The listing builds one solid part. Answer for the finished solid, in the listing's coordinates (mm). Face numbers are marked on the shaded views. A direction names the side the tool comes from. Coordinates: 2 decimals unless noted, no trailing zeros. Order: outer loops, then holes, each group sorted by start corner. A loop starts at its lowest first (then second) coordinate and runs counter-clockwise, first axis right, second up. Notation, with made-up numbers: (74, 27.25) -> (122, 27.25) arc R16 cw to (122, 56.25) -> close; hole circle Ø6 at (-22, -22.5). An arc over 180 degrees is marked (long way). Write each question's results on one line, items separated by ' | '. Start each with the question number.
(1) The part is cut by section A-A, the plane y = 49.5. Give the vertices of the cut face in (x, z) (3 decimals).
(2) Given pin 1 (4 mm diameter, centred on x = 12, z = 48.5, fed in from -Y); pin 2 (11 mm diameter, centred on y = -19.5, z = 8, fed in from +X) (3 decimals); pin 3 (5 mm diameter, centred on y = -28.5, z = 50.5, fed in from +X); pin 4 (14 mm diameter, centred on y = -17.5, z = 19.5, fed in from -X) (3 decimals), each flat-ended and moving along its own axis, determine where each tip first touches the part or whether it passes through.
(3) Determine the mould class of the marked faces 4, 5 and 6 for opening direction X: +X half, -X half, draft (parallel to the pull), parting line (faces both ways), or undercut.
(4) A tool of negligible diameter and unlimited length cuts with its end or side. For the marked faces 1, 2 and 3, from which of +Z, -Z, +X, -X, +Y, -Y can it reach the whole face along a straight path? Write none if from no direction.
(5) The part is cut by section B-B, the plane z = -3.5. Give the vertices of the cut face in (x, y) (3 decimals).
(6) Straight lines are drawn through the part: L1, parallel to Z at x = 18.5, y = 57.5 (3 decimals); L2, parallel to X at y = 20, z = -2 (3 decimals); L3, parallel to Z at x = 94, y = -18.5 (3 decimals). For each, find the intervals that lie inside material, in ascending order.
```python
from build123d import *

# Parameters (mm, degrees)
F1_DEPTH = 63.5
F2_DEPTH = 25.4
F3_DEPTH = 7.9375


with BuildPart() as f1:
    # F0 (on Front) → F1 (new body, symmetric)
    with BuildSketch(Plane.XZ):
        Polygon((-41.275, 9.525), (-41.275, -9.525), (41.275, -9.525), (41.275, 9.525), (22.225, 9.525), align=None)
    extrude(amount=F1_DEPTH, both=True)

    # F0 (on Front) → F2 (join, symmetric)
    with BuildSketch(Plane.XZ):
        with BuildLine():
            Line((22.225, 9.525), (41.275, 9.525))
            Line((41.275, 9.525), (41.275, 27.0002))
            ThreePointArc((41.275, 27.0002), (45.92468, 38.22552), (57.15, 42.8752))
            Line((57.15, 42.8752), (60.325, 42.8752))
            Line((60.325, 42.8752), (60.325, 61.9252))
            Line((60.325, 61.9252), (57.15, 61.9252))
            add(Edge.make_bspline(
                [(56.334677, 61.915682), (56.607115, 61.919454), (56.878897, 61.922626), (57.15, 61.9252)],
                knots=[110.772816, 110.772816, 110.772816, 110.772816, 111.504536, 111.504536, 111.504536, 111.504536], degree=3))
            ThreePointArc((56.334677, 61.915682), (32.167698, 51.405942), (22.225, 27.0002))
            Line((22.225, 27.0002), (22.225, 9.525))
        make_face()
        Polygon((85.725, 61.9252), (60.325, 61.9252), (60.325, 42.8752), (85.725, 42.8752), (85.725, 52.3875), align=None)
    extrude(amount=F2_DEPTH, both=True)

    # F0 (on Front) → F3 (join, symmetric)
    with BuildSketch(Plane.XZ):
        with BuildLine():
            add(Edge.make_bspline(
                [(-41.275, 9.525), (-41.221754, 47.019336), (15.091041, 61.344656), (56.334677, 61.915682)],
                knots=[0, 0, 0, 0, 110.772816, 110.772816, 110.772816, 110.772816], degree=3))
            Line((-41.275, 9.525), (22.225, 9.525))
            Line((22.225, 9.525), (22.225, 27.0002))
            ThreePointArc((22.225, 27.0002), (32.167698, 51.405942), (56.334677, 61.915682))
        make_face()
    extrude(amount=F3_DEPTH, both=True)

    # F0 (on Front) → F4 (revolve)
    with BuildSketch(Plane.XZ):
        Polygon((85.725, 66.675), (85.725, 61.9252), (85.725, 52.3875), (85.725, 42.8752), (85.725, 38.1), (111.125, 38.1), (111.125, 66.675), align=None)
    revolve(axis=Axis((85.725, 0, 45.24375), (0, 0, -1)))


solid = f1.part
```
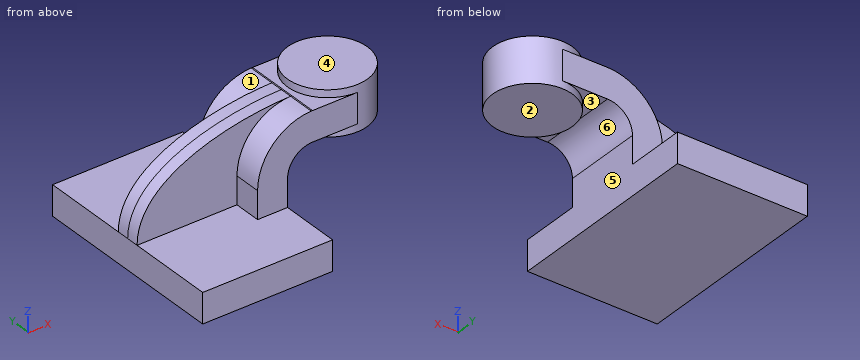
Established:
1) outline: (-41.275, -9.525) -> (41.275, -9.525) -> (41.275, 9.525) -> (-41.275, 9.525) -> close
2) pin 1: stops at y = -7.94 | pin 2: stops at x = 41.275 | pin 3: passes through | pin 4: stops at x = 22.225
3) face 4: draft | face 5: +X half | face 6: undercut
4) face 1: +Z, -X, +Y | face 2: -Z, +X, +Y, -Y | face 3: -Z
5) outline: (-41.275, -63.5) -> (41.275, -63.5) -> (41.275, 63.5) -> (-41.275, 63.5) -> close
6) L1: z = -9.525 to 9.525 | L2: x = -41.275 to 41.275 | L3: z = 38.1 to 66.675
